from build123d import *

# Parameters (mm, degrees)
SKETCH_1_W          = 50
SKETCH_1_H          = 21
EXTRUDE_1_DEPTH     = 34
SKETCH_2_R          = 2
CUT_EXTRUDE_1_DEPTH = 49.548944376
SKETCH_3_R          = 1.5
CUT_EXTRUDE_2_DEPTH = 66.053823869


with BuildPart() as part:
    # 草图1 → 凸台-拉伸1 (new body)
    with BuildSketch(Plane.XY):
        with Locations((0, -13.5)):
            Rectangle(SKETCH_1_W, SKETCH_1_H)
    extrude(amount=EXTRUDE_1_DEPTH)

    # 草图2 → 切除-拉伸1 (cut, through all)
    with BuildSketch(Plane(origin=(0, 0, 0), x_dir=(-1, 0, 0), z_dir=(0, 0, -1))):
        with Locations((-15, -16)):
            Circle(SKETCH_2_R)
        with Locations((15, -16)):
            Circle(SKETCH_2_R)
    extrude(amount=-CUT_EXTRUDE_1_DEPTH, mode=Mode.SUBTRACT)

    # 草图3 → 切除-拉伸2 (cut, through all)
    with BuildSketch(Plane.ZY.offset(25)):
        with Locations(Location((8.252553912, -7, 0), (0, 0, 270))):
            Circle(SKETCH_3_R)
        with Locations(Location((26.252553912, -7, 0), (0, 0, 270))):
            Circle(SKETCH_3_R)
    extrude(amount=-CUT_EXTRUDE_2_DEPTH, mode=Mode.SUBTRACT)


solid = part.part
Source: CAD feature listing. Evaluate the final solid. Frame: model axes, mm. Coordinates: 2 decimals unless noted, no trailing zeros. Write each loop counter-clockwise with the first axis right and the second up, starting at its lowest first coordinate (ties: lowest second). Pieces come first, ordered by that corner, then holes. Notation, with made-up numbers: M -4.5,85 L 48.5,85 A27 cw 48.5,104 Z; hole C -4,-9.75 d7. An arc over 180 degrees is marked long. Use a Markdown table: item, result.
1) Section A-A, the plane x = -15. Output: boundary loops of the cut face in (y, z).
Conclusion:
| item | result |
|---|---|
| outline | M -24,0 L -18,0 L -18,34 L -24,34 Z; M -14,0 L -3,0 L -3,34 L -14,34 Z; hole C -7,8.25 d3; hole C -7,26.25 d3 |
2) Section C-C, the plane z = 29. Output: boundary loops of the cut face in (x, y), then the cut area to 3 significant figures.
Conclusion:
| item | result |
|---|---|
| outline | M -25,-24 L 25,-24 L 25,-3 L -25,-3 Z; hole C -15,-16 d4; hole C 15,-16 d4 |
| area | 1,020 mm^2 |
3) Section B-B, the plane y = -16. Output: boundary loops of the cut face in (x, z), then the cut area to 3 significant figures.
Conclusion:
| item | result |
|---|---|
| outline | M -25,0 L -17,0 L -17,34 L -25,34 Z; M -13,0 L 13,0 L 13,34 L -13,34 Z; M 17,0 L 25,0 L 25,34 L 17,34 Z |
| area | 1,430 mm^2 |
4) Ray query, L1, parallel to Z at x = -9, y = -7; L2, parallel to Y at x = 15, z = 14; L3, parallel to X at y = -17, z = 4.5. Return the intervals inside material, ascending.
Conclusion:
| item | result |
|---|---|
| L1 | z = 0 to 6.75, 9.75 to 24.75, 27.75 to 34 |
| L2 | y = -24 to -18, -14 to -3 |
| L3 | x = -25 to -16.73, -13.27 to 13.27, 16.73 to 25 |
5) Mould query, pull axis X, two halves, no side actions, for faces 1 (the cylindrical face through (15, -14, 17)), 2 (the cylindrical face through (-15, -14, 17)), 3 (the flat face through (-25, -14, 17)), 4 (the flat face through (25, -14, 17)). Classes: pulls with the +X half, pulls with the -X half, needs draft (parallel to the pull), parting line crosses it, or undercut.
Conclusion:
| item | result |
|---|---|
| face 1 | undercut |
| face 2 | undercut |
| face 3 | pulls with the -X half |
| face 4 | pulls with the +X half |
6) Section D-D, the plane x = 7. Output: boundary loops of the cut face in (y, z), then the cut area to 3 significant figures.
Conclusion:
| item | result |
|---|---|
| outline | M -24,0 L -3,0 L -3,34 L -24,34 Z; hole C -7,8.25 d3; hole C -7,26.25 d3 |
| area | 700 mm^2 |
